from build123d import *

# Parameters (mm, degrees)
SKETCH_1_W                  = 80
SKETCH_1_H                  = 80
EXTRUDE_1_DEPTH             = 9
SKETCH_2_W                  = 23.25
SKETCH_2_H                  = 2.5
CUT_EXTRUDE_1_DEPTH         = 90.894382472
SKETCH_10_W                 = 15
SKETCH_10_H                 = 0.5
CUT_EXTRUDE_3_DEPTH         = 90.894382472
HOLE_WIZARD_1_D             = 4.5
HOLE_WIZARD_1_CBORE_D       = 8
HOLE_WIZARD_1_CBORE_DEPTH   = 4.4
HOLE_WIZARD_M3_1_D          = 2.5
HOLE_WIZARD_M3_1_DEPTH      = 7.5
HOLE_WIZARD_M3_1_TIP        = 0.751075774
HOLE_WIZARD_M3_2_D          = 2.5
HOLE_WIZARD_M3_2_DEPTH      = 7.5
HOLE_WIZARD_M3_2_TIP        = 0.751075774
SKETCH_5_OUTSIDE_W          = 104.698
SKETCH_5_OUTSIDE_H          = 104.698
SKETCH_5_OUTSIDE_W_2        = 10
SKETCH_5_OUTSIDE_H_2        = 10
CUT_EXTRUDE_2_DEPTH         = 0.2
HOLE_WIZARD_M3_3_AT_2_COUNT = 2
HOLE_WIZARD_M3_3_AT_2_PITCH = 15


with BuildPart() as part:
    # 草图1 → 凸台-拉伸1 (new body)
    with BuildSketch(Plane(origin=(0, 0, 0), x_dir=(1, 0, 0), z_dir=(0, 1, 0))):
        Rectangle(SKETCH_1_W, SKETCH_1_H)
    extrude(amount=EXTRUDE_1_DEPTH)

    # 草图2 → 切除-拉伸1 (cut, through all)
    with BuildSketch(Plane.XY.offset(40)):
        with Locations((28.375, 7.75)):
            Rectangle(SKETCH_2_W, SKETCH_2_H)
        with Locations((-28.375, 7.75)):
            Rectangle(SKETCH_2_W, SKETCH_2_H)
    extrude(amount=-CUT_EXTRUDE_1_DEPTH, mode=Mode.SUBTRACT)

    # 草图10 → 切除-拉伸3 (cut, through all)
    with BuildSketch(Plane.XY.offset(40)):
        with Locations((32.5, 6.25)):
            Rectangle(SKETCH_10_W, SKETCH_10_H)
        with Locations((-32.5, 6.25)):
            Rectangle(SKETCH_10_W, SKETCH_10_H)
    extrude(amount=-CUT_EXTRUDE_3_DEPTH, mode=Mode.SUBTRACT)

    # 打孔尺寸根据内六角圆柱头螺钉的类型1 (through all)
    with Locations(Plane(origin=(-39.335611713, 6, 5.280516917), x_dir=(1, 0, 0), z_dir=(0, 1, 0))):
        with Locations((4.335611713, 40.280516917), (74.335611713, 40.280516917), (74.335611713, -29.719483083), (4.335611713, -29.719483083)):
            CounterBoreHole(HOLE_WIZARD_1_D / 2, HOLE_WIZARD_1_CBORE_D / 2, HOLE_WIZARD_1_CBORE_DEPTH)

    # M3 螺纹孔1
    with Locations(Plane.ZY.offset(40)):
        with Locations((7, 3), (-13, 3)):
            Hole(HOLE_WIZARD_M3_1_D / 2, depth=HOLE_WIZARD_M3_1_DEPTH)
            with Locations((0, 0, -(HOLE_WIZARD_M3_1_DEPTH + HOLE_WIZARD_M3_1_TIP / 2))):  # 118° drill point
                Cone(0, HOLE_WIZARD_M3_1_D / 2, HOLE_WIZARD_M3_1_TIP, mode=Mode.SUBTRACT)

    # M3 螺纹孔2
    with Locations(Plane(origin=(40, 0, 0), x_dir=(0, 0, -1), z_dir=(1, 0, 0))):
        with Locations((3, 3), (-17, 3)):
            Hole(HOLE_WIZARD_M3_2_D / 2, depth=HOLE_WIZARD_M3_2_DEPTH)
            with Locations((0, 0, -(HOLE_WIZARD_M3_2_DEPTH + HOLE_WIZARD_M3_2_TIP / 2))):  # 118° drill point
                Cone(0, HOLE_WIZARD_M3_2_D / 2, HOLE_WIZARD_M3_2_TIP, mode=Mode.SUBTRACT)

    # 草图5 outside → 切除-拉伸2 (cut)
    with BuildSketch(Plane.XZ):
        Rectangle(SKETCH_5_OUTSIDE_W, SKETCH_5_OUTSIDE_H)
        with Locations((35, 35)):
            Rectangle(SKETCH_5_OUTSIDE_W_2, SKETCH_5_OUTSIDE_H_2, mode=Mode.SUBTRACT)
        with Locations((-35, 35)):
            Rectangle(SKETCH_5_OUTSIDE_W_2, SKETCH_5_OUTSIDE_H_2, mode=Mode.SUBTRACT)
        with Locations((35, -35)):
            Rectangle(SKETCH_5_OUTSIDE_W_2, SKETCH_5_OUTSIDE_H_2, mode=Mode.SUBTRACT)
        with Locations((-35, -35)):
            Rectangle(SKETCH_5_OUTSIDE_W_2, SKETCH_5_OUTSIDE_H_2, mode=Mode.SUBTRACT)
    extrude(amount=-CUT_EXTRUDE_2_DEPTH, mode=Mode.SUBTRACT)

    # 草图11 → M3 螺纹孔3 (revolve, cut)
    with BuildSketch(Plane(origin=(-7.5, 3.7, 40), x_dir=(0, -1, 0), z_dir=(1, 0, 0))):
        Polygon((0, 0), (0, 8.251075774), (1.25, 7.5), (1.25, 0), align=None)
    hole_wizard_m3_3 = revolve(axis=Axis((-7.5, 3.7, 46.35), (0, 0, -1)), mode=Mode.SUBTRACT)

    # M3 螺纹孔3 at 2: M3 螺纹孔3 ×2
    with Locations(*[(i * HOLE_WIZARD_M3_3_AT_2_PITCH, 0, 0) for i in range(1, HOLE_WIZARD_M3_3_AT_2_COUNT)]):
        add(hole_wizard_m3_3, mode=Mode.SUBTRACT)

    # 镜向1: M3 螺纹孔3 across plane
    add(hole_wizard_m3_3.mirror(Plane.XY), mode=Mode.SUBTRACT)

    # 镜向1 copy 1 sketch → 镜向1 copy 1 (revolve, cut)
    with BuildSketch(Plane(origin=(7.5, 3.7, -40), x_dir=(0, -1, 0), z_dir=(1, 0, 0))):
        Polygon((0, 0), (0, -8.251075774), (1.25, -7.5), (1.25, 0), align=None)
    revolve(axis=Axis((7.5, 3.7, -46.35), (0, 0, -1)), mode=Mode.SUBTRACT)


solid = part.part
The listing builds one solid part. Answer for the finished solid, in the listing's coordinates (mm). A direction names the side the tool comes from. Round coordinates to 2 decimals unless told otherwise and drop trailing zeros. Order: outer loops, then holes, each group sorted by start corner. A loop starts at its lowest first (then second) coordinate and runs counter-clockwise, first axis right, second up. Notation, with made-up numbers: (48.5, 56) -> (75.5, 56) arc R22 cw to (75.5, 71) -> close; hole circle Ø10 at (34.5, 9). An arc over 180 degrees is marked (long way). Write each question's results on one line, items separated by ' | '. Start each with the question number.
Q1. Find section B-B (x = 35). Determine the outline of the cut face in (y, z).
Q2. Find section A-A (z = 35). Give the number of separate pieces and of enclosed holes in the cut face, then the cut area to 3 significant figures.
Q3. Find section D-D (x = -20.5). Determine the outline of the cut face in (y, z), then the cut area to 3 significant figures.
Q4. Which of the six approach directions +Z, -Z, +X, -X, +Y, -Y give full straight-line access (tool end or side, diameter ignored) to faces 1 (the flat face through (-21, 6.5, 1)), 2 (the cylindrical face through (-6.74, 4.69, -36.3)), 3 (the flat face through (-33, 1.6, 37)), 4 (the cylindrical face through (36.2, 3.38, -1.81))?
Q5. Each of these flat-tipped pins is pushed along its axis until it touches: pin 1 (1.5 mm diameter, centred on x = 29, z = -7.5, fed in from -Y); pin 2 (2 mm diameter, centred on y = 3, z = 7, fed in from -X); pin 3 (2 mm diameter, centred on x = 7.5, y = 3.7, fed in from +Z). Where does it stop, or does it pass through?
Q6. The mould has two halves that part along Y. Classify faces 5 (the conical face through (7.32, 3.58, -31.88)), 6 (the flat face through (-16.75, 8, 1)), 7 (the flat face through (21, 6.5, 1)): pulls with the +Y half, pulls with the -Y half, needs draft (parallel to the pull), parting line crosses it, or undercut.
Q7. Straight lines are drawn through the part: probe 1 along X at (y, z) = (3.85, 35); probe 2 along Z at (x, y) = (35, 2.95); probe 3 along Y at (x, z) = (36, -3). For each, find the intervals that lie inside material, in ascending order. Write a range as from..to.
Q8. Find section C-C (z = 2). Determine the outline of the cut face in (x, y).
Worked answers:
1) outline: (0, -40) -> (6, -40) -> (6, -39) -> (1.6, -39) -> (1.6, -37.25) -> (0, -37.25) -> close; (0, -32.75) -> (1.6, -32.75) -> (1.6, -31) -> (6, -31) -> (6, 31) -> (1.6, 31) -> (1.6, 32.75) -> (0, 32.75) -> (0, 30) -> (0.2, 30) -> (0.2, -30) -> (0, -30) -> close; (0, 37.25) -> (1.6, 37.25) -> (1.6, 39) -> (6, 39) -> (6, 40) -> (0, 40) -> close; hole circle Ø2.5 at (3, -3); hole circle Ø2.5 at (3, 17)
2) separate pieces: 3 | enclosed holes: 2 | area: 482 mm2
3) outline: (0.2, -40) -> (6.5, -40) -> (6.5, 40) -> (0.2, 40) -> close | area: 504 mm2
4) face 1: +Z, -Z, -X, +Y | face 2: -Z | face 3: +Y | face 4: +X
5) pin 1: stops at y = 0.2 | pin 2: stops at x = -32.35 | pin 3: stops at z = 32.35
6) face 5: undercut | face 6: needs draft | face 7: pulls with the +Y half
7) probe 1: x = -40..-39, -31..-8.74, -6.26..6.26, 8.74..31, 39..40 | probe 2: z = -40..-39, -31..-4.25, -1.75..15.75, 18.25..31, 39..40 | probe 3: y = 0.2..1.75, 4.25..6
8) outline: (-40, 0.2) -> (40, 0.2) -> (40, 6) -> (25, 6) -> (25, 6.5) -> (16.75, 6.5) -> (16.75, 9) -> (-16.75, 9) -> (-16.75, 6.5) -> (-25, 6.5) -> (-25, 6) -> (-40, 6) -> close
